Check sheet for the modelled part. Datum: model origin and axes. Units: mm. A direction names the side the tool comes from. Give positions to 0.01 mm unless a question says otherwise; leave off trailing zeros. Order: outer loops, then holes, each group sorted by start corner. A loop starts at its lowest first (then second) coordinate and runs counter-clockwise, first axis right, second up.
```python
from build123d import *

# Parameters (mm, degrees)
F0_W     = 609.6
F0_H     = 609.6
F1_DEPTH = 508
F2_R     = 76.2
F3_DEPTH = 609.6
F4_R     = 76.2
F5_DEPTH = 609.6
F6_R     = 76.2
F7_DEPTH = 609.6
F8_R     = 76.2
F9_DEPTH = 609.6


with BuildPart() as f1:
    # F0 (on Top) → F1 (new body)
    with BuildSketch(Plane.XY):
        with Locations((207.229508, 194.311477)):
            Rectangle(F0_W, F0_H)
    extrude(amount=F1_DEPTH)

    # F2 (on face) → F3 (join)
    with BuildSketch(Plane.XZ.offset(110.488523)):
        with Locations((209.300384, 170.041427)):
            Circle(F2_R)
    extrude(amount=F3_DEPTH)

    # F4 (on face) → F5 (join)
    with BuildSketch(Plane(origin=(-97.570492, 0, 0), x_dir=(0, -1, 0), z_dir=(-1, 0, 0))):
        with Locations((-183.056265, 169.941157)):
            Circle(F4_R)
    extrude(amount=F5_DEPTH)

    # F6 (on face) → F7 (join)
    with BuildSketch(Plane(origin=(0, 499.111477, 0), x_dir=(-1, 0, 0), z_dir=(0, 1, 0))):
        with Locations((-210.818216, 169.941157)):
            Circle(F6_R)
    extrude(amount=F7_DEPTH)

    # F8 (on face) → F9 (join)
    with BuildSketch(Plane.YZ.offset(512.029508)):
        with Locations((180.434614, 169.941157)):
            Circle(F8_R)
    extrude(amount=F9_DEPTH)


solid = f1.part
```
(1) Go/stop test with flat-tipped pins: P1, Ø2, axis at y = -300, z = 134.5, coming from the +X side; P2, Ø8, axis at y = -33, z = 327, coming from the -X side; P3, Ø4, axis at x = 561, z = 228.5, coming from the -Y side. Record where each tip stops, or that it passes through.
(2) Sectioned sample at A-A (x = 160.5). Enter the section's corners in (y, z), plus the area to 3 significant figures.
(3) Sectioned sample at D-D (x = 411.5). Enter the section's corners in (y, z), plus the area to 3 significant figures.
(4) Sectioned sample at C-C (y = 583). Enter the section's corners in (x, z), plus the area to 3 significant figures.
(5) Thickness scan on L1, parallel to Y at x = 443.5, z = 33.5; L2, parallel to X at y = 273.5, z = 429; L3, parallel to Y at x = 987.5, z = 183. Record the ranges inside material, lowest first.
(6) Sectioned sample at B-B (z = 336.5). Enter the section's corners in (x, y), plus the area to 3 significant figures.
(7) Tool access check on faces 1 (the face through (212, 1108.711, 171)), 2 (the face through (220.738, 799.644, 245.493)), 3 (the face through (-398.1, 239.22, 221.44)), 4 (the face through (812.562, 221.399, 234.193)), 5 (the face through (199.381, -411.021, 245.593)). Record the directions out of +Z, -Z, +X, -X, +Y, -Y that give a thin tool (end or side, any length) a straight path to the whole face; none if there is none.
Values follow:
1. P1: stops at x = 277.22
1. P2: stops at x = -97.57
1. P3: stops at y = 129.37
2. outline: (-720.09, 111.52) - (-110.49, 111.52) - (-110.49, 0) - (499.11, 0) - (499.11, 112.72) - (1108.71, 112.72) - (1108.71, 227.16) - (499.11, 227.16) - (499.11, 508) - (-110.49, 508) - (-110.49, 228.56) - (-720.09, 228.56) - close
2. area: 451,000 mm2
3. outline: (-110.49, 0) - (499.11, 0) - (499.11, 508) - (-110.49, 508) - close
3. area: 310,000 mm2
4. outline: circle Ø152.4 at (210.82, 169.94)
4. area: 18,200 mm2
5. L1: y = -110.49 to 499.11
5. L2: x = -97.57 to 512.03
5. L3: y = 105.36 to 255.51
6. outline: (-97.57, -110.49) - (512.03, -110.49) - (512.03, 499.11) - (-97.57, 499.11) - close
6. area: 372,000 mm2
7. face 1: +Z, -Z, +X, -X, +Y
7. face 2: +Y
7. face 3: -X
7. face 4: +X
7. face 5: -Y
